Verification items for the finished model (mm, model axes). Give positions to 0.01 mm unless a question says otherwise; leave off trailing zeros. Order: outer loops, then holes, each group sorted by start corner. A loop starts at its lowest first (then second) coordinate and runs counter-clockwise, first axis right, second up.
Autodesk Inventor part; units mm, degrees
ref_plane "YZ Plane" through (0, 0, 0) normal (1, 0, 0) x (0, 1, 0)
ref_plane "XZ Plane" through (0, 0, 0) normal (0, 1, 0) x (-1, 0, 0)
ref_plane "XY Plane" through (0, 0, 0) normal (0, 0, 1) x (1, 0, 0)
sketch "Sketch1" plane through (0, 0, 0) normal (0, 1, 0) x (-1, 0, 0)
  point P0 (0, 0)
sketch "Sketch2" plane through (0, 0, 0) normal (0, 1, 0) x (-1, 0, 0)
  line L0 (0, 0) -> (-5, 0)
  line L1 (-5, 0) -> (-5, -4)
  line L2 (-5, -4) -> (0, -4)
  line L3 (0, -4) -> (0, 0)
  line L4 (0, 0) -> (-10, 0)
  line L5 (-10, 0) -> (-10, -15)
  line L6 (-10, -15) -> (0, -15)
  line L7 (0, -15) -> (0, 0)
  circle A0 centre (-2, -2) radius 2
  point P0 (-2, 0)
  point P1 (0, -2)
  point P2 (-2, -4)
  dimension "d0" = 5
  dimension "d1" = 4
  dimension "d2" = 10
  dimension "d3" = 15
sketch "Sketch3" plane through (0, 0, 0) normal (0, 1, 0) x (-1, 0, 0)
  line L0 (0, 0) -> (0, -4.0004)
  line L1 (0, -4.0004) -> (0, -2.0004)
  line L2 (0, -4.0004) -> (-2.5, -4.0004)
  dimension "d4" = 2
  dimension "d5" = 2.5
extrude "Extrusion1" add sketch "Sketch2" along normal blind 50 contours L3 A0 L0 | L3 L2 A0 | L1 L2 L7 L6 L5 L4
sketch "Sketch4" plane through (5, 0, 0) normal (0, 0, 1) x (1, 0, 0)
  line L0 (-5, 0) -> (-5, 50)
  line L1 (-5, 50) -> (5, 50)
  line L2 (5, 50) -> (5, 0)
  line L3 (5, 0) -> (-5, 0)
  line L4 (-5, 0) -> (-5, 50)
extrude "Extrusion2" add sketch "Sketch4" along normal blind 3
sketch "Sketch5" plane through (0, 0, 0) normal (0, -1, 0) x (1, 0, 0)
  arc A0 (2, 0) -> (0, -2) centre (2, -2) ccw
  line L0 (0, -3.5296) -> (0, -0.4704)
  line L1 (0, -0.4704) -> (1.4533, -0.4704)
  line L2 (1.4533, -0.4704) -> (1.4533, -3.5296)
  line L3 (1.4533, -3.5296) -> (0, -3.5296)
  line L4 (0, -3.5296) -> (0, -0.4704)
  point P0 (0, 0)
  point P1 (0.7115, -0.4704)
extrude "Extrusion3" cut sketch "Sketch5" against normal blind 200 contours L1 L2 L3 L0 A0
sketch "Sketch6" plane through (0, 0, 0) normal (0, -1, 0) x (1, 0, 0)
  line L0 (0, -2) -> (0, 3)
  line L1 (0, -0.4704) -> (1.2121, -0.4704)
  line L2 (1.2121, -0.4704) -> (1.2121, -2.1829)
  line L3 (1.2121, -2.1829) -> (0, -2.1829)
  line L4 (0, -2.1829) -> (0, -0.4704)
  point P0 (0, 0)
extrude "Extrusion4" cut sketch "Sketch6" against normal blind 200
sketch "Sketch7" plane through (0, 50, 0) normal (0, 1, 0) x (1, 0, 0)
  point P0 (0, 0)
extrude "Extrusion5" add sketch "Sketch2" against normal blind 50 contours L1 L2 L7 L6 L5 L4
sketch "Sketch8" plane through (0, 0, 0) normal (0, -1, 0) x (1, 0, 0)
  line L0 (5, 0) -> (10, 0)
  line L1 (0, -0.4704) -> (0, 3)
  line L2 (10, 0) -> (0, 0)
  line L3 (0, 0) -> (0, 3)
  line L4 (0, 3) -> (10, 3)
  line L5 (10, 3) -> (10, 0)
extrude "Extrusion6" add sketch "Sketch8" along normal blind 50
sketch "Sketch9" plane through (0, 0, 0) normal (0, -1, 0) x (1, 0, 0)
  point P0 (0, 0)
properties part number "basebody"
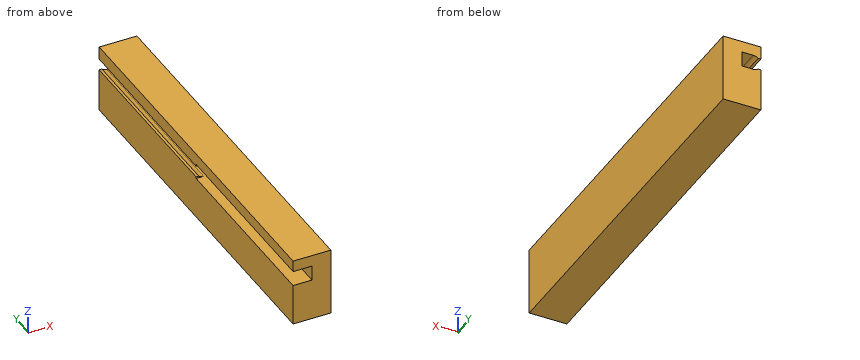
(1) Scan lines: line 1 (Z direction, x = 3, y = 29); line 2 (X direction, y = -26, z = -1.5). Record each from-to range of solid material in increasing order.
Solved:
line 1: z = -15 to -4, 0 to 3
line 2: x = 5 to 10
(2) Section check B-B, the plane y = 3.5. Enter the section's corners in (x, z).
Solved:
outline: (0, -15) - (10, -15) - (10, 3) - (0, 3) - (0, -0.47) - (0.71, -0.47) arc R2 cw to (2, 0) - (5, 0) - (5, -4) - (2, -4) arc R2 cw to (0.71, -3.53) - (0, -3.53) - close
(3) Go/stop test with flat-tipped pins: pin 1 (2 mm diameter, centred on y = 24, z = -1, fed in from -X); pin 2 (0.5 mm diameter, centred on x = 0.5, z = -0.5, fed in from -Y). Record where each tip stops, or that it passes through.
Solved:
pin 1: stops at x = 0
pin 2: stops at y = 0
(4) Section check A-A, the plane y = -18. Enter the section's corners in (x, z).
Solved:
outline: (0, -15) - (10, -15) - (10, 3) - (0, 3) - (0, 0) - (5, 0) - (5, -4) - (0, -4) - close
